from build123d import *

# Parameters (mm, degrees)
F0_W        = 111.2626455724
F0_H        = 92.8305797279
F0_R        = 35.6593077027
F1_DEPTH    = 25
F2_T1_DEPTH = 312.2046894127
F2_T3_DEPTH = 330.6367552572


# Not quite as in the source:
# - a fillet or chamfer that OpenCascade refuses, or shapes differently, is made with other operations: its cross-section is extruded or revolved along the edge and cut away or added


with BuildPart() as f1:
    # F0 (on Front) → F1 (new body)
    with BuildSketch(Plane.XZ):
        with Locations((1.6756337136, -1.5080738813)):
            Rectangle(F0_W, F0_H)
        Circle(F0_R, mode=Mode.SUBTRACT)
    extrude(amount=F1_DEPTH)

    # F2: fillet of radius 51 on 2 edges, made by hand

    # F2_s2 → F2_t1 (cut)
    with BuildSketch(Plane.XY.offset(-157.6104185876)):
        with BuildLine():
            ThreePointArc((57.3069564998, 0), (38.6808969088, -18.3113980822), (13.4321345628, -25))
            Line((13.4321345628, -25), (57.3069564998, -25))
            Line((57.3069564998, -25), (57.3069564998, 0))
        make_face()
    extrude(amount=F2_T1_DEPTH, mode=Mode.SUBTRACT)

    # F2_s4 → F2_t3 (cut)
    with BuildSketch(Plane.YZ.offset(-163.642743915)):
        with BuildLine():
            ThreePointArc((0, 44.9072159827), (-18.3113980822, 26.2811563916), (-25, 1.0323940457))
            Line((-25, 1.0323940457), (-25, 44.9072159827))
            Line((-25, 44.9072159827), (0, 44.9072159827))
        make_face()
    extrude(amount=F2_T3_DEPTH, mode=Mode.SUBTRACT)


solid = f1.part
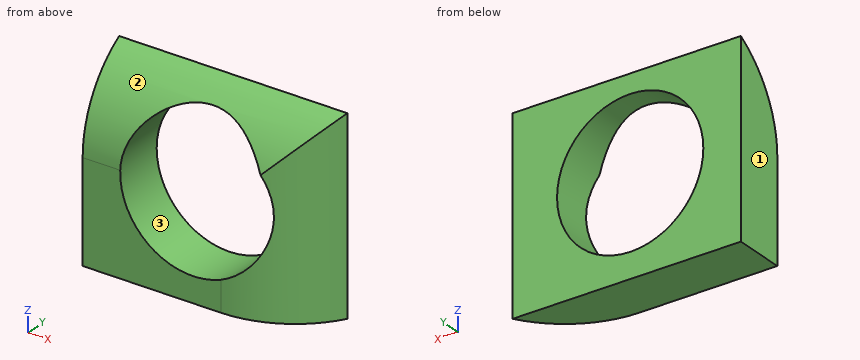
Could you check a few things on this model? Use its own coordinates, in mm. Face numbers are marked on the shaded views. Give positions to 0.01 mm unless a question says otherwise; leave off trailing zeros. Order: outer loops, then holes, each group sorted by start corner. A loop starts at its lowest first (then second) coordinate and runs counter-clockwise, first axis right, second up. Notation, with made-up numbers: (-16, -9) -> (19, -9) arc R19 ccw to (19, 8) -> close; hole circle Ø5 at (-6.75, -4.75). An arc over 180 degrees is marked (long way). Answer in a Markdown table with one row per item. Add a question column.
Item 1: Imagine slicing it at A-A (x = 0). List the corners of the cut face in (y, z) for me, and give its area (3 significant figures).
Item 2: Imagine slicing it at D-D (y = -11.75). List the corners of the cut face in (x, z) for me.
Item 3: We'd pull the mould along Z, two halves only. Please class the marked faces 1, 2 and 3: pulls with the +Z half, pulls with the -Z half, needs draft (parallel to the pull), parting line crosses it, or undercut.
Item 4: I'm going to push flat-ended pins straight in: P1, Ø1, axis at x = -13, z = -33, coming from the +Y side; P2, Ø6, axis at x = 39, z = -2.5, coming from the -Y side (3 decimals); P3, Ø8, axis at x = -11, y = -14, coming from the +Z side; P4, Ø12, axis at y = -18, z = -37.5, coming from the +X side. Where does each tip first touch, or does it pass through?
Item 5: Please list where these lines run through material, in increasing order: probe 1 along Z at (x, y) = (0, -19); probe 2 along Z at (x, y) = (-30.5, -20.75); probe 3 along X at (y, z) = (-15.25, -6).
Item 6: Imagine slicing it at B-B (z = 5.5). List the corners of the cut face in (x, y) for me, and give its area (3 significant figures).
Item 7: Imagine slicing it at C-C (y = -18.25). List the corners of the cut face in (x, z) for me.
Result:
| question | item | result |
|---|---|---|
| 1 | outline | (-25, -47.92) -> (0, -47.92) -> (0, -35.66) -> (-25, -35.66) -> close; (-11.44, 35.66) -> (0, 35.66) -> (0, 44.91) arc R51 ccw to start |
| 1 | area | 365 mm2 |
| 2 | outline | (-53.96, -47.92) -> (47.72, -47.92) -> (47.72, 35.32) -> (4.88, 35.32) arc R35.66 cw (long way) to (-4.88, 35.32) -> (-53.96, 35.32) -> close |
| 3 | face 1 | needs draft |
| 3 | face 2 | pulls with the +Z half |
| 3 | face 3 | undercut |
| 4 | P1 | y = 0 |
| 4 | P2 | y = -19.735 |
| 4 | P3 | z = 37.16 |
| 4 | P4 | x = 47.45 |
| 5 | probe 1 | -47.92 to -35.66 |
| 5 | probe 2 | -47.92 to -18.48, 18.48 to 21.41 |
| 5 | probe 3 | -53.96 to -35.15, 35.15 to 43.42 |
| 6 | outline | (-53.96, -24.8) -> (-35.23, -24.8) -> (-35.23, 0) -> (-53.96, 0) -> close; (35.23, -20.11) arc R51 ccw to (57.31, 0) -> (35.23, 0) -> close |
| 6 | area | 731 mm2 |
| 7 | outline | (-53.96, -47.92) -> (38.79, -47.92) -> (38.79, 26.39) -> (23.98, 26.39) arc R35.66 cw (long way) to (-23.98, 26.39) -> (-53.96, 26.39) -> close |
